```python
from build123d import *

# Parameters (mm, degrees)
SKETCH3_W                           = 82
SKETCH3_H                           = 54
BOSS_EXTRUDE2_DEPTH                 = 20
MOTOR_START                         = -5
SKETCH6_W                           = 42.2
SKETCH6_H                           = 42.2
MOTOR_POCKET_DEPTH                  = 73.781745931
SKETCH7_R                           = 11
MOTOR_PILOT_HOLE_DEPTH              = 78.781745931
M3_CLEARANCE_HOLE1_MOTOR_MOUNTING_D = 3.4
SKETCH12_R                          = 7.95
CUT_EXTRUDE4_DEPTH                  = 78.781745931
SKETCH14_R                          = 11.1
SLEEVE_BEARING_RECESS_DEPTH         = 3.5
SKETCH15_R                          = 7.5
CUT_EXTRUDE7_DEPTH                  = 84.886828525
BOSS_EXTRUDE8_START                 = 27
BOSS_EXTRUDE8_DEPTH                 = 12
MIRROR6_START                       = 27
MIRROR6_COPY_1_DEPTH                = 12
M4_CLEARANCE_HOLE1_AT_2_COUNT       = 2
M4_CLEARANCE_HOLE1_AT_2_PITCH       = 23.872983346
CLAMP_START                         = -5
CLAMP_NUT_POCKETS_DEPTH             = 3.5
MIRROR8_START                       = -5
MIRROR8_COPY_3_DEPTH                = 3.5
CHAMFER3_SIZE                       = 8
FILLET8_R                           = 3


with BuildPart() as part:
    # Sketch3 → Boss-Extrude2 (new, symmetric)
    with BuildSketch(Plane(origin=(0, 0, 0), x_dir=(1, 0, 0), z_dir=(0, 1, 0))):
        with Locations((-20, 0)):
            Rectangle(SKETCH3_W, SKETCH3_H)
    extrude(amount=BOSS_EXTRUDE2_DEPTH, both=True)

    # Sketch6 → Motor Pocket (cut, through all)
    with BuildSketch(Plane(origin=(0, 20, 0), x_dir=(1, 0, 0), z_dir=(0, 1, 0)).offset(MOTOR_START)):
        Rectangle(SKETCH6_W, SKETCH6_H)
    extrude(amount=-MOTOR_POCKET_DEPTH, mode=Mode.SUBTRACT)

    # Sketch7 → Motor Pilot Hole (cut, through all)
    with BuildSketch(Plane(origin=(0, 20, 0), x_dir=(1, 0, 0), z_dir=(0, 1, 0))):
        with Locations(Location((0, 0, 0), (0, 0, 270))):
            Circle(SKETCH7_R)
    extrude(amount=-MOTOR_PILOT_HOLE_DEPTH, mode=Mode.SUBTRACT)

    # M3 Clearance Hole1 - Motor Mounting (through all)
    with Locations(Plane(origin=(0, 20, 0), x_dir=(-1, 0, 0), z_dir=(0, 1, 0))):
        with Locations((15.490941809, 15.490941809), (-15.490941809, -15.490941809), (15.490941809, -15.490941809), (-15.490941809, 15.490941809)):
            Hole(M3_CLEARANCE_HOLE1_MOTOR_MOUNTING_D / 2)

    # Sketch12 → Cut-Extrude4 (cut, through all)
    with BuildSketch(Plane(origin=(0, 20, 0), x_dir=(1, 0, 0), z_dir=(0, 1, 0))):
        with Locations(Location((-40, 0, 0), (0, 0, 270))):
            Circle(SKETCH12_R)
    extrude(amount=-CUT_EXTRUDE4_DEPTH, mode=Mode.SUBTRACT)

    # Sketch14 → Sleeve Bearing Recess (cut)
    with BuildSketch(Plane.XZ.offset(20)):
        with Locations(Location((-40, 0, 0), (0, 0, 270))):
            Circle(SKETCH14_R)
    extrude(amount=-SLEEVE_BEARING_RECESS_DEPTH, mode=Mode.SUBTRACT)

    # Sketch15 → Cut-Extrude7 (cut, through all)
    with BuildSketch(Plane.XY.offset(27)):
        Circle(SKETCH15_R)
    extrude(amount=-CUT_EXTRUDE7_DEPTH, mode=Mode.SUBTRACT)

    # Sketch16 → Boss-Extrude8 (add)
    with BuildSketch(Plane.XY.offset(BOSS_EXTRUDE8_START)):
        with BuildLine():
            Line((21, 20), (21, -20))
            Line((21, -20), (29, -20))
            Line((29, -20), (29, -3.872983346))
            ThreePointArc((29, -3.872983346), (26, 0), (29, 3.872983346))
            Line((29, 3.872983346), (29, 20))
            Line((29, 20), (21, 20))
        make_face()
    boss_extrude8 = extrude(amount=-BOSS_EXTRUDE8_DEPTH)

    # Mirror5: Boss-Extrude8 across plane
    add(boss_extrude8.mirror(Plane.XY))

    # Mirror6: Boss-Extrude8 across plane
    add(boss_extrude8.mirror(Plane(origin=(-20, 0, 0), x_dir=(0, 0, 1), z_dir=(1, 0, 0))))

    # Mirror6 copy 1 sketch → Mirror6 copy 1 (add)
    with BuildSketch(Plane(origin=(-40, 0, 0), x_dir=(-1, 0, 0), z_dir=(0, 0, -1)).offset(MIRROR6_START)):
        with BuildLine():
            Line((21, 20), (21, -20))
            Line((21, -20), (29, -20))
            Line((29, -20), (29, -3.872983346))
            ThreePointArc((29, -3.872983346), (26, 0), (29, 3.872983346))
            Line((29, 3.872983346), (29, 20))
            Line((29, 20), (21, 20))
        make_face()
    extrude(amount=-MIRROR6_COPY_1_DEPTH)

    # Sketch18 → M4 Clearance Hole1 (revolve, cut)
    with BuildSketch(Plane(origin=(29, 11.936491673, 21), x_dir=(0, 0, -1), z_dir=(0, 1, 0))):
        Polygon((0, 0), (0, 13.351936393), (2.25, 12), (2.25, 0), align=None)
    m4_clearance_hole1 = revolve(axis=Axis((35.35, 11.936491673, 21), (-1, 0, 0)), mode=Mode.SUBTRACT)

    # M4 Clearance Hole1 at 2: M4 Clearance Hole1 ×2
    with Locations(*[(0, -i * M4_CLEARANCE_HOLE1_AT_2_PITCH, 0) for i in range(1, M4_CLEARANCE_HOLE1_AT_2_COUNT)]):
        add(m4_clearance_hole1, mode=Mode.SUBTRACT)

    # Sketch17 → Clamp Nut Pockets (cut)
    with BuildSketch(Plane(origin=(29, 0, 0), x_dir=(0, 0, -1), z_dir=(1, 0, 0)).offset(CLAMP_START)):
        Polygon((-21, -7.981642329), (-27, -7.981642329), (-27, -15.891341017), (-21, -15.891341017), (-17.575, -13.913916345), (-17.575, -9.959067001), align=None)
        Polygon((-21, 7.981642329), (-17.575, 9.959067001), (-17.575, 13.913916345), (-21, 15.891341017), (-27, 15.891341017), (-27, 7.981642329), align=None)
    clamp_nut_pockets = extrude(amount=-CLAMP_NUT_POCKETS_DEPTH, mode=Mode.SUBTRACT)

    # Mirror7: M4 Clearance Hole1, Clamp Nut Pockets across plane
    add(m4_clearance_hole1.mirror(Plane.XY), mode=Mode.SUBTRACT)
    add(clamp_nut_pockets.mirror(Plane.XY), mode=Mode.SUBTRACT)

    # Mirror7 copy 1 sketch → Mirror7 copy 1 (revolve, cut)
    with BuildSketch(Plane(origin=(29, -11.936491673, -21), x_dir=(0, 0, 1), z_dir=(0, 1, 0))):
        Polygon((0, 0), (0, -13.351936393), (2.25, -12), (2.25, 0), align=None)
    revolve(axis=Axis((35.35, -11.936491673, -21), (1, 0, 0)), mode=Mode.SUBTRACT)

    # Mirror8: M4 Clearance Hole1, Clamp Nut Pockets across plane
    add(m4_clearance_hole1.mirror(Plane(origin=(-20, 0, 0), x_dir=(0, 0, 1), z_dir=(1, 0, 0))), mode=Mode.SUBTRACT)
    add(clamp_nut_pockets.mirror(Plane(origin=(-20, 0, 0), x_dir=(0, 0, 1), z_dir=(1, 0, 0))), mode=Mode.SUBTRACT)

    # Mirror8 copy 1 sketch → Mirror8 copy 1 (revolve, cut)
    with BuildSketch(Plane(origin=(-69, -11.936491673, 21), x_dir=(0, 0, -1), z_dir=(0, 1, 0))):
        Polygon((0, 0), (0, -13.351936393), (2.25, -12), (2.25, 0), align=None)
    revolve(axis=Axis((-75.35, -11.936491673, 21), (-1, 0, 0)), mode=Mode.SUBTRACT)

    # Mirror8 copy 2 sketch → Mirror8 copy 2 (revolve, cut)
    with BuildSketch(Plane(origin=(-69, 11.936491673, -21), x_dir=(0, 0, 1), z_dir=(0, 1, 0))):
        Polygon((0, 0), (0, 13.351936393), (2.25, 12), (2.25, 0), align=None)
    revolve(axis=Axis((-75.35, 11.936491673, -21), (1, 0, 0)), mode=Mode.SUBTRACT)

    # Mirror8 copy 3 sketch → Mirror8 copy 3 (cut)
    with BuildSketch(Plane.ZY.offset(69).offset(MIRROR8_START)):
        Polygon((-21, -7.981642329), (-27, -7.981642329), (-27, -15.891341017), (-21, -15.891341017), (-17.575, -13.913916345), (-17.575, -9.959067001), align=None)
        Polygon((-21, 7.981642329), (-17.575, 9.959067001), (-17.575, 13.913916345), (-21, 15.891341017), (-27, 15.891341017), (-27, 7.981642329), align=None)
    extrude(amount=-MIRROR8_COPY_3_DEPTH, mode=Mode.SUBTRACT)

    # Mirror8 copy 4 sketch → Mirror8 copy 4 (revolve, cut)
    with BuildSketch(Plane(origin=(-69, -11.936491673, -21), x_dir=(0, 0, 1), z_dir=(0, 1, 0))):
        Polygon((0, 0), (0, 13.351936393), (2.25, 12), (2.25, 0), align=None)
    revolve(axis=Axis((-75.35, -11.936491673, -21), (1, 0, 0)), mode=Mode.SUBTRACT)

    # Chamfer3
    # the kernel refuses this chamfer: 8 mm, written as the material it adds along each edge
    with BuildSketch(Plane(origin=(-61, 20, -15), x_dir=(-0.9996219169112968, 0, -0.027495876610586296), z_dir=(0, -1, 0))) as chamfer3_piece_1_section:
        Polygon((CHAMFER3_SIZE * 0.999621916911, -CHAMFER3_SIZE * 0.0274958766106), (-CHAMFER3_SIZE * 0.0274958766106, -CHAMFER3_SIZE * 0.999621916911), (0, 0), align=None)
    chamfer3_piece_1 = extrude(amount=40, mode=Mode.PRIVATE)
    chamfer3_piece_1 = chamfer3_piece_1 - Plane(origin=(-70, 0, -12.302715733), x_dir=(0.2500000000000009, -0.968245836551854, 0), z_dir=(0, 0, -1)) * Cylinder(4, 112, mode=Mode.PRIVATE)
    add(chamfer3_piece_1)
    with BuildSketch(Plane(origin=(-61, 20, 15), x_dir=(0.027495876610586487, 0, -0.9996219169112968), z_dir=(0, -1, 0))) as chamfer3_piece_2_section:
        Polygon((CHAMFER3_SIZE * 0.999621916911, -CHAMFER3_SIZE * 0.0274958766106), (-CHAMFER3_SIZE * 0.0274958766106, -CHAMFER3_SIZE * 0.999621916911), (0, 0), align=None)
    chamfer3_piece_2 = extrude(amount=40, mode=Mode.PRIVATE)
    chamfer3_piece_2 = chamfer3_piece_2 - Plane(origin=(-70, 0, 12.302715733), x_dir=(0.2500000000000009, -0.968245836551854, 0), z_dir=(0, 0, 1)) * Cylinder(4, 112, mode=Mode.PRIVATE)
    add(chamfer3_piece_2)
    with BuildSketch(Plane(origin=(21, 20, 15), x_dir=(0.9996219169112968, 0, 0.02749587661058627), z_dir=(0, -1, 0))) as chamfer3_piece_3:
        Polygon((CHAMFER3_SIZE * 0.999621916911, -CHAMFER3_SIZE * 0.0274958766106), (-CHAMFER3_SIZE * 0.0274958766106, -CHAMFER3_SIZE * 0.999621916911), (0, 0), align=None)
    extrude(amount=5)
    with BuildSketch(Plane(origin=(21, 20, -15), x_dir=(0.9996219169112968, 0, -0.02749587661058627), z_dir=(0, -1, 0))) as chamfer3_piece_4:
        Polygon((CHAMFER3_SIZE * 0.999621916911, CHAMFER3_SIZE * 0.0274958766106), (-CHAMFER3_SIZE * 0.0274958766106, CHAMFER3_SIZE * 0.999621916911), (0, 0), align=None)
    extrude(amount=5)

    # Fillet8
    fillet8_edges = [part.edges().sort_by_distance(p)[0] for p in [
        (-61, 0, -7),
        (-61, 0, 7),
        (21, 17.5, 7),
        (21, 17.5, -7),
    ]]
    fillet(fillet8_edges, radius=FILLET8_R)


solid = part.part
```
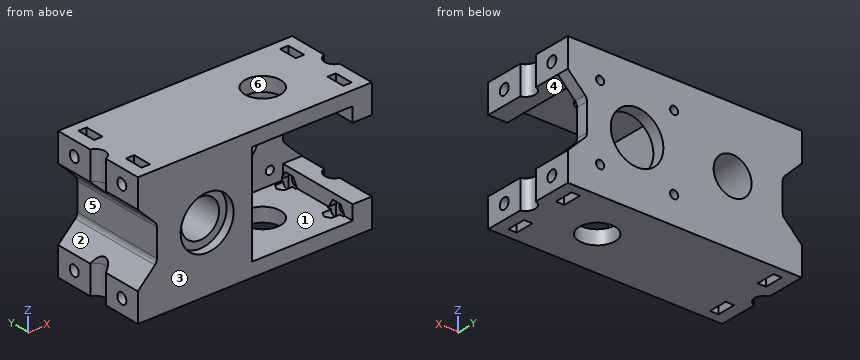
For this review, take the finished solid that the model builds, in its own axes (mm). Face numbers are marked on the shaded views. A direction names the side the tool comes from. Give positions to 0.01 mm unless a question says otherwise; leave off trailing zeros. Order: outer loops, then holes, each group sorted by start corner. A loop starts at its lowest first (then second) coordinate and runs counter-clockwise, first axis right, second up.
1) Take a section at A-A (y = 0). Give the boundary of the cut face in (x, z), then the cut area to 3 significant figures.
2) Insertion check: pin 1 (2.5 mm diameter, centred on y = -11.94, z = -21, fed in from -X); pin 2 (1.8 mm diameter, centred on x = -63, y = -12, fed in from -Z) (3 decimals); pin 3 (2.5 mm diameter, centred on y = -12.5, z = 20.5, fed in from -X); pin 4 (3 mm diameter, centred on x = 15.49, z = 15.49, fed in from -Y). Each pin has a flat end and moves straight along its axis. Give the tip position at first contact, or say it passes through.
3) Take a section at B-B (z = 0). Give the boundary of the cut face in (x, y), then the cut area to 3 significant figures.
4) Take a section at D-D (z = 10). Give the boundary of the cut face in (x, y).
5) The part is to be moulded in two halves that separate along X. For the marked faces 4, 5 and 6, say which applies: released by +X, released by -X, zero draft, split by the parting line, or undercut.
6) Wall thickness on line 1 (Y direction, x = -59, z = -21); line 2 (X direction, y = 14, z = -23); line 3 (Y direction, x = 26.6, z = -21): over which ranges is each line inside the solid? List them lowest first.
7) For the marked faces 1, 2 and 3, list the 3-axis set-ups (+Z, -Z, +X, -X, +Y, -Y) from which the entire face can be reached by the end or side of a thin tool; tool diameter is ignored.
8) Take a section at C-C (x = -40). Give the boundary of the cut face in (y, z).
Derived:
1. outline: (-66, -27) - (-7.5, -27) - (-7.5, -21.1) - (-21.1, -21.1) - (-21.1, 21.1) - (-7.5, 21.1) - (-7.5, 27) - (-66, 27) - (-66, 12) - (-61.88, 7.88) arc R3 cw to (-61, 5.76) - (-61, -5.76) arc R3 cw to (-61.88, -7.88) - (-66, -12) - close; (7.5, -27) - (26, -27) - (26, -15) - (21, -15) - (21, -21.1) - (7.5, -21.1) - close; (7.5, 21.1) - (21, 21.1) - (21, 15) - (26, 15) - (26, 27) - (7.5, 27) - close; hole circle Ø15.9 at (-40, 0)
1. area: 2,570 mm2
2. pin 1: stops at x = -56.4
2. pin 2: stops at z = -17.575
2. pin 3: stops at x = -56.85
2. pin 4: passes through
3. outline: (-61, -20) - (-51.1, -20) - (-51.1, -16.5) - (-47.95, -16.5) - (-47.95, 20) - (-61, 20) - close; (-32.05, -16.5) - (-28.9, -16.5) - (-28.9, -20) - (-21.1, -20) - (-21.1, 15) - (-11, 15) - (-11, 20) - (-32.05, 20) - close; (11, 15) - (21, 15) - (21, 20) - (11, 20) - close
3. area: 1,040 mm2
4. outline: (-64, -20) - (-44.82, -20) - (-44.82, -16.5) - (-35.18, -16.5) - (-35.18, -20) - (-21.1, -20) - (-21.1, 15) - (-4.58, 15) - (-4.58, 20) - (-64, 20) - close; (4.58, 15) - (24, 15) - (24, 20) - (4.58, 20) - close
5. face 4: zero draft
5. face 5: released by -X
5. face 6: undercut
6. line 1: y = -20 to -14.19, -9.69 to 9.69, 14.19 to 20
6. line 2: x = -69 to -64, -60.5 to 20.5, 24 to 29
6. line 3: y = -20 to -14.19, -9.69 to -2.11, 2.11 to 9.69, 14.19 to 20
7. face 1: -Y
7. face 2: -X, +Y, -Y
7. face 3: +Z, -Z, +X, -X, -Y
8. outline: (-20, -27) - (20, -27) - (20, -7.95) - (-16.5, -7.95) - (-16.5, -11.1) - (-20, -11.1) - close; (-20, 11.1) - (-16.5, 11.1) - (-16.5, 7.95) - (20, 7.95) - (20, 27) - (-20, 27) - close
